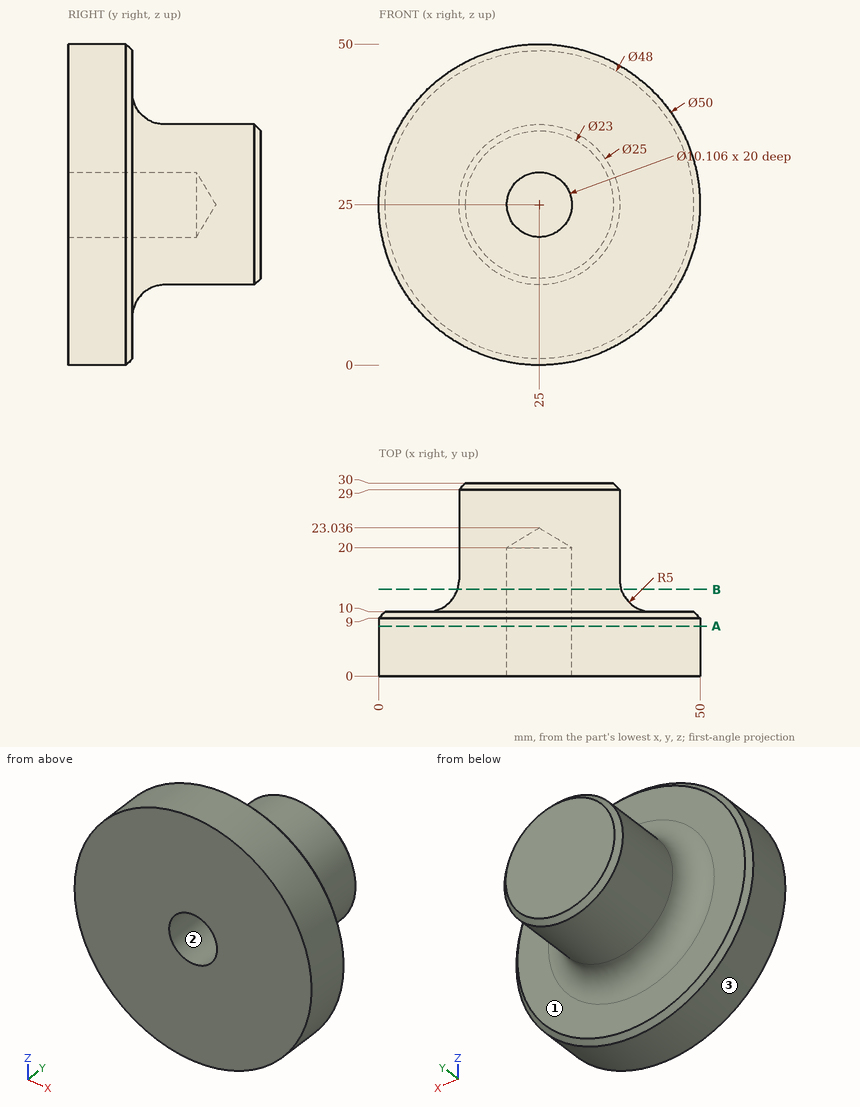
Source: three-view drawing plus pictorial views. Frame: mm from the lowest corner of the part. A direction names the side the tool comes from. Round coordinates to 2 decimals unless told otherwise and drop trailing zeros. Loops run counter-clockwise (first coordinate to the right, second up) from the corner with the lowest first, then second, coordinate; pieces in that order, holes last. Notation, with made-up numbers: (-39, 20) - (-14, 20) arc R29 ccw to (-14, 45) - close; hole circle Ø2 at (41.5, 77). An arc over 180 degrees is marked (long way). Write item = value, one per line. Start each with the question number.
Item 1: Section query A-A on y = 7.75. Output: boundary loops of the cut face in (x, z).
Item 2: Reachability of the marked faces 1, 2 and 3 from +Z, -Z, +X, -X, +Y, -Y: full face, straight path, thin tool, end or side. Return the list, or none.
Item 3: Section query B-B on y = 13.5. Output: boundary loops of the cut face in (x, z), plus the area to 3 significant figures.
Item 4: Material intervals for line 1 (Z direction, x = 25, y = 5.25); line 2 (Y direction, x = 35.5, z = 7); line 3 (Z direction, x = 25, y = 11), sorted ascending.
Item 5: First-contact query: pin 1 Ø8 at (x, z) = (25, 25) entering from -Y; pin 2 Ø5 at (y, z) = (15, 12) entering from +X; pin 3 Ø2 at (x, z) = (30.5, 19) entering from -Y; pin 4 Ø2 at (y, z) = (26, 22.5) entering from +X. Flat tips, straight axial feed; report the tip coordinate or a pass-through.
Results list:
q1.outline = circle Ø50 at (25, 25); hole circle Ø10.11 at (25, 25)
q2.face_1 = +Y
q2.face_2 = -Y
q2.face_3 = +Y, -Y
q3.outline = circle Ø25.46 at (25, 25); hole circle Ø10.11 at (25, 25)
q3.area = 429 mm²
q4.line_1 = 0 to 19.95, 30.05 to 50
q4.line_2 = 0 to 10
q4.line_3 = 10.5 to 19.95, 30.05 to 39.5
q5.pin_1 = 20.63
q5.pin_2 = 31.78
q5.pin_3 = 0
q5.pin_4 = 37.41
